Read the model definition and answer for the solid it produces. Units are mm, in the model's axes. Coordinates: 2 decimals unless noted, no trailing zeros. Loops run counter-clockwise (first coordinate to the right, second up) from the corner with the lowest first, then second, coordinate; pieces in that order, holes last. Notation, with made-up numbers: (-18.75, -24) - (2.25, -24) arc R22 ccw to (2.25, 12) - close; hole circle Ø7 at (82.5, -25.5). An arc over 180 degrees is marked (long way). One line per item, written item: value. Start each with the question number.
from build123d import *
from OCP.BRepFilletAPI import BRepFilletAPI_MakeChamfer

# Parameters (mm, degrees)
SKETCH_1_W                          = 2.54
SKETCH_1_H                          = 2.54
EXTRUDE_1_DEPTH                     = 8.51
SKETCH_4_W                          = 0.7
SKETCH_4_H                          = 0.7
CUT_EXTRUDE_1_DEPTH                 = 8.21
CHAMFER_3_SIZE                      = 0.4
SKETCH_2_W                          = 0.5
SKETCH_2_H                          = 0.5
EXTRUDE_2_DEPTH                     = 3.15
CHAMFER_2_SIZE                      = 0.5
CHAMFER_2_SIZE2                     = 0.106278281
PATTERN_LINEAR_1_COUNT              = 3
PATTERN_LINEAR_1_PITCH              = 2.54
CHAMFER_3_OF_PATTERN_LINEAR_1_SIZE  = 0.4
CHAMFER_2_OF_PATTERN_LINEAR_1_SIZE  = 0.5
CHAMFER_2_OF_PATTERN_LINEAR_1_SIZE2 = 0.106278281


with BuildPart() as part:
    # Эскиз1 → Бобышка-Вытянуть1 (new body)
    with BuildSketch(Plane(origin=(0, 0, 0), x_dir=(-1, 0, 0), z_dir=(0, 1, 0))):
        Rectangle(SKETCH_1_W, SKETCH_1_H)
    extrude_1 = extrude(amount=EXTRUDE_1_DEPTH)

    # Эскиз4 → Вырез-Вытянуть1 (cut)
    with BuildSketch(Plane(origin=(0, 8.51, 0), x_dir=(1, 0, 0), z_dir=(0, 1, 0))):
        Rectangle(SKETCH_4_W, SKETCH_4_H)
    cut_extrude_1 = extrude(amount=-CUT_EXTRUDE_1_DEPTH, mode=Mode.SUBTRACT)

    # Фаска3
    chamfer_3_edges = [part.edges().sort_by_distance(p)[0] for p in [
        (-0.35, 8.51, 0),
        (0, 8.51, 0.35),
        (0.35, 8.51, 0),
        (0, 8.51, -0.35),
    ]]
    chamfer(chamfer_3_edges, length=CHAMFER_3_SIZE)

    # Эскиз2 → Бобышка-Вытянуть2 (add)
    with BuildSketch(Plane(origin=(0, 0, 0), x_dir=(-1, 0, 0), z_dir=(0, 1, 0))):
        Rectangle(SKETCH_2_W, SKETCH_2_H)
    extrude_2 = extrude(amount=-EXTRUDE_2_DEPTH)

    # Фаска2: one chamfer whose edges measure the first distance from different faces: ONE call of the kernel's chamfer builder (chamfer() names one face for all edges)
    chamfer_2_edges_1 = [part.edges().sort_by_distance(p)[0] for p in [
        (-0.25, -3.15, 0),
    ]]
    chamfer_2_side_1 = [part.faces().sort_by_distance(p)[0] for p in [
        (-0.25, -1.575, 0),
    ]]
    chamfer_2_edges_2 = [part.edges().sort_by_distance(p)[0] for p in [
        (0.25, -3.15, 0),
    ]]
    chamfer_2_side_2 = [part.faces().sort_by_distance(p)[0] for p in [
        (0.25, -1.575, 0),
    ]]
    chamfer_2 = BRepFilletAPI_MakeChamfer(part.part.solid().wrapped)
    for e in chamfer_2_edges_1:
        chamfer_2.Add(CHAMFER_2_SIZE, CHAMFER_2_SIZE2, e.wrapped, chamfer_2_side_1[0].wrapped)  # the first distance lies on this face
    for e in chamfer_2_edges_2:
        chamfer_2.Add(CHAMFER_2_SIZE, CHAMFER_2_SIZE2, e.wrapped, chamfer_2_side_2[0].wrapped)  # the first distance lies on this face
    add(Compound.cast(chamfer_2.Shape()), mode=Mode.REPLACE)

    # Линейный массив1: Бобышка-Вытянуть1, Вырез-Вытянуть1, Бобышка-Вытянуть2 ×3
    with Locations(*[(0, 0, -i * PATTERN_LINEAR_1_PITCH) for i in range(1, PATTERN_LINEAR_1_COUNT)]):
        add(extrude_1)
        add(cut_extrude_1, mode=Mode.SUBTRACT)
        add(extrude_2)

    # Фаска3 of Линейный массив1
    chamfer_3_of_pattern_linear_1_edges = [part.edges().sort_by_distance(p)[0] for p in [
        (-0.35, 8.51, -2.54),
        (0, 8.51, -2.19),
        (0.35, 8.51, -2.54),
        (0, 8.51, -2.89),
        (-0.35, 8.51, -5.08),
        (0, 8.51, -4.73),
        (0.35, 8.51, -5.08),
        (0, 8.51, -5.43),
    ]]
    chamfer(chamfer_3_of_pattern_linear_1_edges, length=CHAMFER_3_OF_PATTERN_LINEAR_1_SIZE)

    # Фаска2 of Линейный массив1: one chamfer whose edges measure the first distance from different faces: ONE call of the kernel's chamfer builder (chamfer() names one face for all edges)
    chamfer_2_of_pattern_linear_1_edges_1 = [part.edges().sort_by_distance(p)[0] for p in [
        (-0.25, -3.15, -2.54),
    ]]
    chamfer_2_of_pattern_linear_1_side_1 = [part.faces().sort_by_distance(p)[0] for p in [
        (-0.25, -1.575, -2.54),
    ]]
    chamfer_2_of_pattern_linear_1_edges_2 = [part.edges().sort_by_distance(p)[0] for p in [
        (0.25, -3.15, -2.54),
    ]]
    chamfer_2_of_pattern_linear_1_side_2 = [part.faces().sort_by_distance(p)[0] for p in [
        (0.25, -1.575, -2.54),
    ]]
    chamfer_2_of_pattern_linear_1_edges_3 = [part.edges().sort_by_distance(p)[0] for p in [
        (-0.25, -3.15, -5.08),
    ]]
    chamfer_2_of_pattern_linear_1_side_3 = [part.faces().sort_by_distance(p)[0] for p in [
        (-0.25, -1.575, -5.08),
    ]]
    chamfer_2_of_pattern_linear_1_edges_4 = [part.edges().sort_by_distance(p)[0] for p in [
        (0.25, -3.15, -5.08),
    ]]
    chamfer_2_of_pattern_linear_1_side_4 = [part.faces().sort_by_distance(p)[0] for p in [
        (0.25, -1.575, -5.08),
    ]]
    chamfer_2_of_pattern_linear_1 = BRepFilletAPI_MakeChamfer(part.part.solid().wrapped)
    for e in chamfer_2_of_pattern_linear_1_edges_1:
        chamfer_2_of_pattern_linear_1.Add(CHAMFER_2_OF_PATTERN_LINEAR_1_SIZE, CHAMFER_2_OF_PATTERN_LINEAR_1_SIZE2, e.wrapped, chamfer_2_of_pattern_linear_1_side_1[0].wrapped)  # the first distance lies on this face
    for e in chamfer_2_of_pattern_linear_1_edges_2:
        chamfer_2_of_pattern_linear_1.Add(CHAMFER_2_OF_PATTERN_LINEAR_1_SIZE, CHAMFER_2_OF_PATTERN_LINEAR_1_SIZE2, e.wrapped, chamfer_2_of_pattern_linear_1_side_2[0].wrapped)  # the first distance lies on this face
    for e in chamfer_2_of_pattern_linear_1_edges_3:
        chamfer_2_of_pattern_linear_1.Add(CHAMFER_2_OF_PATTERN_LINEAR_1_SIZE, CHAMFER_2_OF_PATTERN_LINEAR_1_SIZE2, e.wrapped, chamfer_2_of_pattern_linear_1_side_3[0].wrapped)  # the first distance lies on this face
    for e in chamfer_2_of_pattern_linear_1_edges_4:
        chamfer_2_of_pattern_linear_1.Add(CHAMFER_2_OF_PATTERN_LINEAR_1_SIZE, CHAMFER_2_OF_PATTERN_LINEAR_1_SIZE2, e.wrapped, chamfer_2_of_pattern_linear_1_side_4[0].wrapped)  # the first distance lies on this face
    add(Compound.cast(chamfer_2_of_pattern_linear_1.Shape()), mode=Mode.REPLACE)


solid = part.part
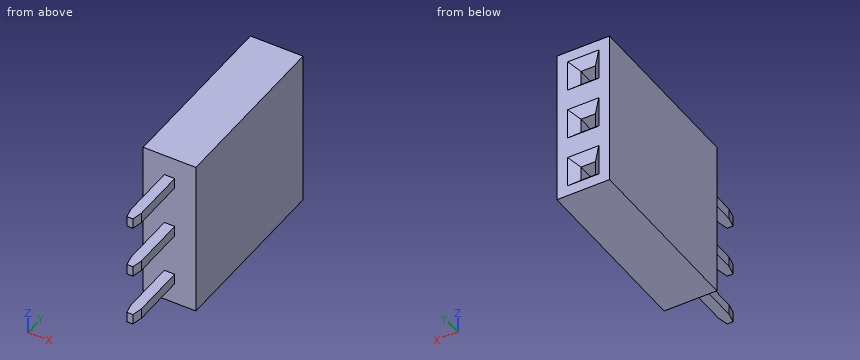
1) Section A-A, the plane y = 2.25 is taken. Determine the outline of the cut face in (x, z), and give its area (3 significant figures).
2) Straight lines are drawn through the part: L1, parallel to Z at x = -0.2, y = 1.75; L2, parallel to Z at x = -0.2, y = -1.5. For each, find the intervals that lie inside material, in ascending order.
3) Section B-B, the plane y = -2.25 is taken. Determine the outline of the cut face in (x, z), and give its area (3 significant figures).
4) Section C-C, the plane z = 0 is taken. Determine the outline of the cut face in (x, y), and give its area (3 significant figures).
5) Flat-ended cylindrical pins translate along their axes: P1, Ø0.8, axis at x = 0.5, z = -4, coming from the -Y side; P2, Ø0.6, axis at y = -1, z = 0, coming from the -X side. Find the tip coordinate at first contact, or state that the pin passes through.
Answer below:
1. outline: (-1.27, -6.35) - (1.27, -6.35) - (1.27, 1.27) - (-1.27, 1.27) - close; hole (-0.35, -5.43) - (0.35, -5.43) - (0.35, -4.73) - (-0.35, -4.73) - close; hole (-0.35, -2.89) - (0.35, -2.89) - (0.35, -2.19) - (-0.35, -2.19) - close; hole (-0.35, -0.35) - (0.35, -0.35) - (0.35, 0.35) - (-0.35, 0.35) - close
1. area: 17.9 mm2
2. L1: -6.35 to -5.43, -4.73 to -2.89, -2.19 to -0.35, 0.35 to 1.27
2. L2: -5.33 to -4.83, -2.79 to -2.29, -0.25 to 0.25
3. outline: (-0.25, -5.33) - (0.25, -5.33) - (0.25, -4.83) - (-0.25, -4.83) - close; (-0.25, -2.79) - (0.25, -2.79) - (0.25, -2.29) - (-0.25, -2.29) - close; (-0.25, -0.25) - (0.25, -0.25) - (0.25, 0.25) - (-0.25, 0.25) - close
3. area: 0.750 mm2
4. outline: (-1.27, 0) - (-0.25, 0) - (-0.25, -2.65) - (-0.14, -3.15) - (0.14, -3.15) - (0.25, -2.65) - (0.25, 0) - (1.27, 0) - (1.27, 8.51) - (0.75, 8.51) - (0.35, 8.11) - (0.35, 0.3) - (-0.35, 0.3) - (-0.35, 8.11) - (-0.75, 8.51) - (-1.27, 8.51) - close
4. area: 17.2 mm2
5. P1: y = 0
5. P2: x = -0.25
